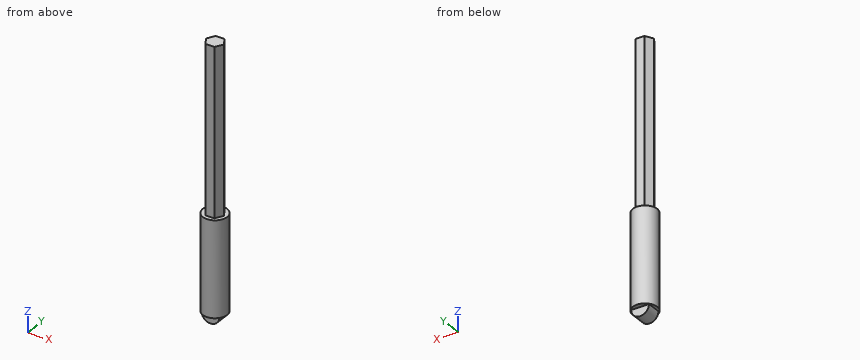
from build123d import *

# Parameters (mm, degrees)
SKETCH1_R                = 1.025
BOSS_EXTRUDE1_DEPTH      = 5
BOSS_EXTRUDE5_DEPTH      = 0.25
BOSS_EXTRUDE5_DEPTH_BACK = 0.2
BOSS_EXTRUDE6_DEPTH      = 0.375
BOSS_EXTRUDE7_START      = 0.375
BOSS_EXTRUDE7_DEPTH      = 0.375
BOSS_EXTRUDE9_DEPTH      = 14
SKETCH7_R                = 1.025
BOSS_EXTRUDE10_DEPTH     = 3
BOSS_EXTRUDE11_DEPTH     = 3


with BuildPart() as part:
    # Sketch1 → Boss-Extrude1 (new body)
    with BuildSketch(Plane.XY):
        Circle(SKETCH1_R)
    extrude(amount=BOSS_EXTRUDE1_DEPTH)

    # Sketch3 → Boss-Extrude5 (add, two sides: drawn at the far end of the back side and taken through both)
    with BuildSketch(Plane(origin=(0, 0, 0), x_dir=(1, 0, 0), z_dir=(0, 1, 0)).offset(-BOSS_EXTRUDE5_DEPTH_BACK)):
        with BuildLine():
            Line((-0.75, 0), (0.75, 0))
            ThreePointArc((0.75, 0), (0, 0.75), (-0.75, 0))
        make_face()
    extrude(amount=BOSS_EXTRUDE5_DEPTH + BOSS_EXTRUDE5_DEPTH_BACK)

    # Sketch5 → Boss-Extrude6 (add)
    with BuildSketch(Plane(origin=(0, 0.25, 0), x_dir=(1, 0, 0), z_dir=(0, 1, 0))):
        with BuildLine():
            Line((-0.75, 0), (0.75, 0))
            ThreePointArc((0.75, 0), (0, 0.75), (-0.75, 0))
        make_face()
    extrude(amount=BOSS_EXTRUDE6_DEPTH)

    # Sketch6 → Boss-Extrude7 (add)
    with BuildSketch(Plane.XZ.offset(0.2).offset(BOSS_EXTRUDE7_START)):
        with BuildLine():
            Line((0.75, 0), (-0.75, 0))
            ThreePointArc((-0.75, 0), (0, -0.75), (0.75, 0))
        make_face()
    extrude(amount=-BOSS_EXTRUDE7_DEPTH)

    # Sketch2 → Boss-Extrude9 (add)
    with BuildSketch(Plane.XY.offset(5)):
        Polygon((0.75055535, 0), (0.375277675, 0.65), (-0.375277675, 0.65), (-0.75055535, 0), (-0.375277675, -0.65), (0.375277675, -0.65), align=None)
    extrude(amount=BOSS_EXTRUDE9_DEPTH)

    # Sketch7 → Boss-Extrude10 (add)
    with BuildSketch(Plane.XY.offset(5)):
        Circle(SKETCH7_R)
    extrude(amount=BOSS_EXTRUDE10_DEPTH)

    # Sketch8 → Boss-Extrude11 (add)
    with BuildSketch(Plane.XY.offset(19)):
        Polygon((0.75055535, 0), (0.375277675, 0.65), (-0.375277675, 0.65), (-0.75055535, 0), (-0.375277675, -0.65), (0.375277675, -0.65), align=None)
    extrude(amount=BOSS_EXTRUDE11_DEPTH)


solid = part.part
Source: CAD feature listing. Evaluate the final solid. Frame: model axes, mm. Round coordinates to 2 decimals unless told otherwise and drop trailing zeros. Loops run counter-clockwise (first coordinate to the right, second up) from the corner with the lowest first, then second, coordinate; pieces in that order, holes last.
Q1. Ray query, line 1 (Z direction, x = 0.35, y = 0.7); line 2 (X direction, y = -0.7, z = 7); line 3 (Y direction, x = 0.5, z = 8.25). Return the intervals inside material, ascending.
Q2. First-contact query: P1, Ø0.6, axis at x = 0.5, y = 0, coming from the -Z side. Flat tip, straight axial feed; report the tip coordinate or a pass-through.
Q3. Section C-C, the plane z = 20. Return loops of the section in (x, y).
Q4. Section A-A, the plane x = 0. Return loops of the section in (y, z) (3 decimals), plus the area to 3 significant figures.
Q5. Section B-B, the plane y = -0.35. Return loops of the section in (x, z), plus the area to 3 significant figures.
Solutions:
1. line 1: z = 0 to 8
1. line 2: x = -0.75 to 0.75
1. line 3: y = -0.43 to 0.43
2. P1: stops at z = -0.72
3. outline: (-0.75, 0) - (-0.38, -0.65) - (0.38, -0.65) - (0.75, 0) - (0.38, 0.65) - (-0.38, 0.65) - close
4. outline: (-1.025, 0) - (-0.575, 0) - (-0.575, -0.75) - (0.625, -0.75) - (0.625, 0) - (1.025, 0) - (1.025, 8) - (0.65, 8) - (0.65, 22) - (-0.65, 22) - (-0.65, 8) - (-1.025, 8) - close
4. area: 35.5 mm2
5. outline: (-0.96, 0) - (-0.75, 0) arc R0.75 ccw to (0.75, 0) - (0.96, 0) - (0.96, 8) - (0.55, 8) - (0.55, 22) - (-0.55, 22) - (-0.55, 8) - (-0.96, 8) - close
5. area: 31.7 mm2
